Design review of the part built by this model. Coordinates are the model's own, in mm. A direction names the side the tool comes from. Give positions to 0.01 mm unless a question says otherwise; leave off trailing zeros. Loops run counter-clockwise (first coordinate to the right, second up) from the corner with the lowest first, then second, coordinate; pieces in that order, holes last. Notation, with made-up numbers: (-16.5, 38) - (41.5, 38) arc R25 ccw to (41.5, 66) - close; hole circle Ø10 at (46, 31). An arc over 180 degrees is marked (long way). One line per item, written item: value. Start each with the question number.
```python
from build123d import *

# Parameters (mm, degrees)
F1_DEPTH = 500
F2_DEPTH = 2


with BuildPart() as f1:
    # F0 (on Right) → F1 (new body, symmetric)
    with BuildSketch(Plane.YZ):
        with BuildLine():
            ThreePointArc((2.4382058168, -7.6193931776), (6.461642459, -4.7166912908), (8, 0))
            ThreePointArc((8, 0), (-4.7166912908, 6.461642459), (-2.4382058168, -7.6193931776))
            Line((-2.4382058168, -7.6193931776), (0, 0))
            Line((0, 0), (2.4382058168, -7.6193931776))
        make_face()
        with BuildLine():
            Line((0, 0), (-2.4382058168, -7.6193931776))
            ThreePointArc((-2.4382058168, -7.6193931776), (0, -8), (2.4382058168, -7.6193931776))
            Line((2.4382058168, -7.6193931776), (0, 0))
        make_face()
        with BuildLine():
            ThreePointArc((2.4382058168, -7.6193931776), (0, -8), (-2.4382058168, -7.6193931776))
            Line((-2.4382058168, -7.6193931776), (-8, -25))
            Line((-8, -25), (0, -25))
            Line((0, -25), (8, -25))
            Line((8, -25), (2.4382058168, -7.6193931776))
        make_face()
        Polygon((0, -25), (-8, -25), (-18, -25), (-18, -30), (18, -30), (18, -25), (8, -25), align=None)
    extrude(amount=F1_DEPTH, both=True)

    # F0 (on Right) → F2 (cut)
    with BuildSketch(Plane.YZ):
        with BuildLine():
            ThreePointArc((2.4382058168, -7.6193931776), (0, -8), (-2.4382058168, -7.6193931776))
            Line((-2.4382058168, -7.6193931776), (-8, -25))
            Line((-8, -25), (0, -25))
            Line((0, -25), (8, -25))
            Line((8, -25), (2.4382058168, -7.6193931776))
        make_face()
        Polygon((0, -25), (-8, -25), (-18, -25), (-18, -30), (18, -30), (18, -25), (8, -25), align=None)
    extrude(amount=F2_DEPTH, mode=Mode.SUBTRACT)


solid = f1.part
```
(1) For pin 1 Ø2 at (x, y) = (357, 13) entering from +Z; pin 2 Ø2 at (x, z) = (389.5, -12) entering from +Y; pin 3 Ø8 at (x, z) = (-373, 1.5) entering from -Y, all flat-tipped, find the tip position at first contact; note any pin that passes through.
(2) Take a section at A-A on x = -344.5. State the section outline as (y, z) points.
(3) Machinability: for faces 5 (the flat face through (-246, 0, -30)), 6 (the flat face through (254.49, -5.18, -16.19)), 7 (the flat face through (-246.5, 5.258, -16.431)), which of the approach directions +Z, -Z, +X, -X, +Y, -Y give a long, thin tool a straight path to every point of the face, cutting with its end or side? Answer none if there is none.
(4) To check wall thickness, follow L1, parallel to X at y = 3, z = -19; L2, parallel to Z at x = -303.5, y = -13; L3, parallel to Z at x = 290.5, y = -1. State the ranges of each line that lie inside material, in increasing order. Write a range as from..to.
(5) Take a section at B-B on z = 0. State the section outline as (x, y) points.
(6) Draft analysis for pull direction X (two halves, no side actions). For faces 1 (the flat face through (2, 0, -24)), 2 (the flat face through (254.486, 5.258, -16.431)), 3 (the flat face through (0, 0, -24)), 4 (the flat face through (-500, 0, -15)), state which applies: pulls with the +X half, pulls with the -X half, needs draft (parallel to the pull), parting line crosses it, or undercut.
Here are the results:
1. pin 1: z = -25
1. pin 2: y = 4.16
1. pin 3: y = -8
2. outline: (-18, -30) - (18, -30) - (18, -25) - (8, -25) - (2.44, -7.62) arc R8 ccw (long way) to (-2.44, -7.62) - (-8, -25) - (-18, -25) - close
3. face 5: -Z, +X, -X, +Y, -Y
3. face 6: +X, -X, -Y
3. face 7: +X, -X, +Y
4. L1: -500..0, 2..500
4. L2: -30..-25
4. L3: -30..7.94
5. outline: (-500, -8) - (500, -8) - (500, 8) - (-500, 8) - close
6. face 1: undercut
6. face 2: needs draft
6. face 3: undercut
6. face 4: pulls with the -X half
